Autodesk Inventor part; units mm, degrees
ref_plane "YZ Plane" through (0, 0, 0) normal (1, 0, 0) x (0, 1, 0)
ref_plane "XZ Plane" through (0, 0, 0) normal (0, 1, 0) x (-1, 0, 0)
ref_plane "XY Plane" through (0, 0, 0) normal (0, 0, 1) x (1, 0, 0)
sketch "Connector Hole Layout" plane through (0, 0, 0) normal (0, 1, 0) x (-1, 0, 0)
  circle A0 centre (42.9488, 7.9638) radius 1.6 construction
  circle A1 centre (-17.5388, 30.2138) radius 1.6 construction
  circle A2 centre (42.9488, 52.4638) radius 1.6 construction
  line L0 (42.9488, 7.9638) -> (42.9488, 52.4638) construction
  line L1 (41.4471, 51.9114) -> (-16.0371, 30.7661) construction
  point P0 (42.9488, 30.2138)
  dimension "d0" = 3.2
  dimension "d22" = 44.5
  dimension "d23" = 61.25
sketch "Sketch8" plane through (0, 0, 0) normal (0, 1, 0) x (-1, 0, 0)
  circle A0 centre (42.9488, 7.9638) radius 1.6 construction
  circle A1 centre (42.9488, 52.4638) radius 1.6 construction
  circle A2 centre (-17.5388, 30.2138) radius 1.6 construction
  circle A3 centre (42.9488, 7.9638) radius 4
  point P0 (0, 0)
  dimension "d51" = 8
extrude "Extrusion5" add sketch "Sketch8" along normal blind 7
sketch "Sketch9" plane through (-42.9488, 7, 7.9638) normal (0, 1, 0) x (1, 0, 0)
  point P0 (42.9488, 7.9638)
  point P1 (0, 0)
hole "Hole2" at (-42.9488, 7, 7.9638) direction (0, -1, 0) diameter 4 depth 5 tip angle 118
chamfer "Chamfer3" distance 1 distance2 2 1 edges at (-38.9488, 7, 7.9638) measured on face at (-46.2385, 7, 7.5643)
pattern_sketch "Sketch Driven Pattern1" from (-42.9488, 0, 7.9638) copies at (-42.9488, 0, 52.4638) at (17.5388, 0, 30.2138)
sketch "Sketch10" plane through (-42.9488, 0, 52.4638) normal (0, -1, 0) x (1, 0, 0)
  circle A0 centre (0, 0) radius 4
  line L0 (1.3809, 3.7541) -> (61.8684, -18.4959)
  circle A1 centre (60.4875, -22.25) radius 4
  line L1 (61.8684, -26.0041) -> (1.3809, -48.2541)
  circle A2 centre (0, -44.5) radius 4
  line L2 (-4, -44.5) -> (-4, 0)
  circle A3 centre (0, 0) radius 4
  circle A4 centre (0, -44.5) radius 4
  point P0 (42.9488, -52.4638)
extrude "Extrusion6" add sketch "Sketch10" along normal blind 4.5
properties part number "db-25_standoffs_plate"
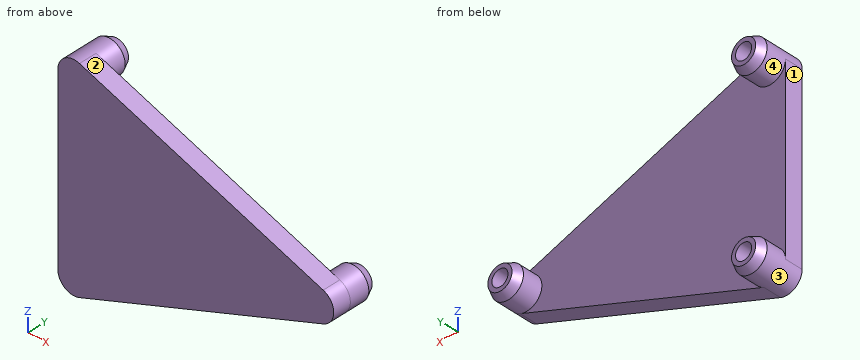
Can you work these out from the model? Positions are in its coordinate system, mm. Face numbers are marked on the shaded views. Give positions to 0.01 mm unless a question says otherwise; leave off trailing zeros. Loops run counter-clockwise (first coordinate to the right, second up) from the corner with the lowest first, then second, coordinate; pieces in that order, holes last. Notation, with made-up numbers: (77.25, 37.5) - (121.25, 37.5) arc R9 cw to (121.25, 49.5) - close; hole circle Ø1 at (81.5, 2.5). An arc over 180 degrees is marked (long way). Return JSON: item names as keys, results as strings.
1. I want a section at B-B on y = 6. Please give me the cut outline in (x, z).
Output values:
{"outline": "circle Ø7 at (-42.95, 7.96); circle Ø7 at (-42.95, 52.46); circle Ø7 at (17.54, 30.21); hole circle Ø4 at (-42.95, 7.96); hole circle Ø4 at (-42.95, 52.46); hole circle Ø4 at (17.54, 30.21)"}
2. I want a section at A-A on y = 2.75. Please give me the cut outline in (x, z), and give its area (3 significant figures).
Output values:
{"outline": "circle Ø8 at (-42.95, 7.96); circle Ø8 at (-42.95, 52.46); circle Ø8 at (17.54, 30.21); hole circle Ø4 at (-42.95, 7.96); hole circle Ø4 at (-42.95, 52.46); hole circle Ø4 at (17.54, 30.21)", "area": "113 mm²"}
3. I'm going to push flat-ended pins straight in: pin 1 Ø5 at (x, y) = (-29.5, 2) entering from -Z; pin 2 Ø5 at (y, z) = (4, 28) entering from +X; pin 3 Ø5 at (x, y) = (-14.5, 1.5) entering from +Z. Where does each tip first touch, or does it pass through?
Output values:
{"pin 1": "stops at z = 8.1", "pin 2": "stops at x = 21.54", "pin 3": "stops at z = 47"}
4. I want a section at D-D on z = 19.5. Please give me the cut outline in (x, y).
Output values:
{"outline": "(-46.95, -4.5) - (0, -4.5) - (0, 0) - (-46.95, 0) - close"}
5. If I drill on line 1 (Y direction, x = -39.5, z = 14); line 2 (Z direction, x = -19.5, y = -1.5); line 3 (Z direction, x = -29.5, y = -1), over which ranges is the centre line in solid material (lowest first)?
Output values:
{"line 1": "y = -4.5 to 0", "line 2": "z = 12.33 to 48.1", "line 3": "z = 8.65 to 51.78"}
6. I want a section at C-C on x = -23. Please give me the cut outline in (y, z).
Output values:
{"outline": "(-4.5, 11.04) - (0, 11.04) - (0, 49.39) - (-4.5, 49.39) - close"}
7. We'd pull the mould along Z, two halves only. Please class the marked faces 1, 2, 3 and 4: +Z half, -Z half, draft (parallel to the pull), parting line (faces both ways), or undercut.
Output values:
{"face 1": "draft", "face 2": "+Z half", "face 3": "undercut", "face 4": "undercut"}
